Here's how the part is built. I have some questions about the finished solid (model axes, mm). A direction names the side the tool comes from. Give positions to 0.01 mm unless a question says otherwise; leave off trailing zeros. Write each loop counter-clockwise with the first axis right and the second up, starting at its lowest first coordinate (ties: lowest second). Pieces come first, ordered by that corner, then holes. Notation, with made-up numbers: (31, 64) -> (55, 64) arc R17 ccw to (55, 80) -> close; hole circle Ø1 at (-20, 34). An arc over 180 degrees is marked (long way). Use CSV: the item, a comma, the result in double quotes. Start each with the question number.
(1) Suppose I cut it at B-B on z = 1.25. List the corners of the cut face in (x, y) for me, plus the area to 3 significant figures.
(2) Which directions (+Z, -Z, +X, -X, +Y, -Y) give clear straight access to the entire face, cutting with the end or side of a thin tool? Please do faces 1 (the flat face through (-11, 3.5, 0)), 2 (the flat face through (12, 4.5, 5)), 3 (the flat face through (-13, 4.5, 0)), 4 (the flat face through (12, 4, 3.5)).
(3) Suppose I cut it at C-C on y = 0.5. List the corners of the cut face in (x, z) for me.
(4) Suppose I cut it at D-D on x = 3. List the corners of the cut face in (y, z) for me, plus the area to 3 significant figures.
(5) For pin 1 Ø3 at (y, z) = (5.5, -2) entering from -X; pin 2 Ø3 at (x, z) = (13, -6) entering from +Y; pin 3 Ø2.5 at (x, z) = (-11, 1.5) entering from -Y; pin 4 Ø1 at (y, z) = (1, 1) entering from +X, each with a flat end and sliding along its axis, tell me the tip position at first contact or that it passes through.
(6) Suppose I cut it at A-A on x = 12.5. List the corners of the cut face in (y, z) for me, plus the area to 3 significant figures.
(7) I need wall thicknesses on L1, parallel to X at y = 5, z = 3.5; L2, parallel to X at y = 1.5, z = -4; L3, parallel to Y at x = -13.5, z = 6.5. Which ranges of each line are inside material? Lowest first, please. Write a range as [from, to].
(8) If we mould it in two halves opening along Z, with no side actions, what happens to faces 5 (the flat face through (0, 5, -7.5)), 6 (the flat face through (15, 4, 6)), 7 (the flat face through (12, 4, -3.5))? For each: pulls with the +Z half, pulls with the -Z half, needs draft (parallel to the pull), parting line crosses it, or undercut.
from build123d import *

# Parameters (mm, degrees)
SKETCH1_W           = 30
SKETCH1_H           = 15
BOSS_EXTRUDE1_DEPTH = 7
SKETCH3_W           = 5
SKETCH3_H           = 2.5
SKETCH3_W_2         = 9
SKETCH3_H_2         = 3.5
SKETCH3_W_3         = 16
CUT_EXTRUDE1_DEPTH  = 18.5
SKETCH4_W           = 5
SKETCH4_H           = 1.5
CUT_EXTRUDE2_DEPTH  = 18.5


with BuildPart() as part:
    # Sketch1 → Boss-Extrude1 (new body)
    with BuildSketch(Plane(origin=(0, 0, 0), x_dir=(1, 0, 0), z_dir=(0, 1, 0))):
        Rectangle(SKETCH1_W, SKETCH1_H)
    extrude(amount=BOSS_EXTRUDE1_DEPTH)

    # Sketch3 → Cut-Extrude1 (cut, symmetric)
    with BuildSketch(Plane.XY.offset(7.5)):
        with Locations((-12.5, 5.75)):
            Rectangle(SKETCH3_W, SKETCH3_H)
        with Locations((-10.5, 1.75)):
            Rectangle(SKETCH3_W_2, SKETCH3_H_2)
        with Locations((12.5, 5.75)):
            Rectangle(SKETCH3_W, SKETCH3_H)
        with Locations((7, 1.75)):
            Rectangle(SKETCH3_W_3, SKETCH3_H_2)
    extrude(amount=CUT_EXTRUDE1_DEPTH, both=True, mode=Mode.SUBTRACT)

    # Sketch4 → Cut-Extrude2 (cut, symmetric)
    with BuildSketch(Plane(origin=(0, 7, 0), x_dir=(1, 0, 0), z_dir=(0, 1, 0))):
        with Locations((12.5, 2.75)):
            Rectangle(SKETCH4_W, SKETCH4_H)
        with Locations((12.5, -2.75)):
            Rectangle(SKETCH4_W, SKETCH4_H)
    extrude(amount=CUT_EXTRUDE2_DEPTH, both=True, mode=Mode.SUBTRACT)


solid = part.part
Geometry says:
1,outline,"(-15, 3.5) -> (-6, 3.5) -> (-6, 0) -> (-1, 0) -> (-1, 3.5) -> (15, 3.5) -> (15, 4.5) -> (10, 4.5) -> (10, 7) -> (-10, 7) -> (-10, 4.5) -> (-15, 4.5) -> close"
1,area,"97.5 mm²"
2,face 1,"+Z, -Z, -X, -Y"
2,face 2,"+Z, -Z, +X, +Y"
2,face 3,"+Z, -Z, -X, +Y"
2,face 4,"+X, +Y, -Y"
3,outline,"(-6, -7.5) -> (-1, -7.5) -> (-1, 7.5) -> (-6, 7.5) -> close"
4,outline,"(3.5, -7.5) -> (7, -7.5) -> (7, 7.5) -> (3.5, 7.5) -> close"
4,area,"52.5 mm²"
5,pin 1,"x = -15"
5,pin 2,"y = 4.5"
5,pin 3,"y = 3.5"
5,pin 4,"x = -1"
6,outline,"(3.5, -7.5) -> (4.5, -7.5) -> (4.5, -3.5) -> (3.5, -3.5) -> close; (3.5, -2) -> (4.5, -2) -> (4.5, 2) -> (3.5, 2) -> close; (3.5, 3.5) -> (4.5, 3.5) -> (4.5, 7.5) -> (3.5, 7.5) -> close"
6,area,"12.0 mm²"
7,L1,"[-10, 10]"
7,L2,"[-6, -1]"
7,L3,"[3.5, 4.5]"
8,face 5,"pulls with the -Z half"
8,face 6,"needs draft"
8,face 7,"undercut"
